Could you check a few things on this model? Use its own coordinates, in mm. Face numbers are marked on the shaded views. A direction names the side the tool comes from. Coordinates: 2 decimals unless noted, no trailing zeros. Loops run counter-clockwise (first coordinate to the right, second up) from the corner with the lowest first, then second, coordinate; pieces in that order, holes last.
1) Thinking about a two-plate mould opening in X: for the marked faces 1, 2, 3 and 4, which applies, released by +X, released by -X, zero draft, split by the parting line, or undercut?
2) For the marked faces 5, 6 and 7, which set-ups out of +Z, -Z, +X, -X, +Y, -Y let a thin tool reach every point of the face, with its end or its side?
3) Imagine slicing it at D-D on x = -197.5. Please give me the cut outline in (y, z), plus the area to 3 significant figures.
4) Imagine slicing it at C-C on y = -66. Please give me the cut outline in (x, z).
5) Imagine slicing it at A-A on y = 0. Please give me the cut outline in (x, z), plus the area to 3 significant figures.
6) Will these pins go through, and if not, where does the flat tip stop? P1, Ø9.5, axis at y = -12, z = 20, coming from the -X side; P2, Ø4, axis at x = -90.5, y = 101, coming from the -Z side; P3, Ø5, axis at y = -100.5, z = -15.5, coming from the +X side; P4, Ø24, axis at x = 0, y = 0, coming from the -Z side.
7) If I drill on line 1 along Z through (x, y) = (47.5, -89); line 2 along Y through (x, z) = (-156, -18); line 3 along X through (y, z) = (-44, 22.5), over which ranges is the centre line in solid material (lowest first)?
8) Imagine slicing it at B-B on x = -27. Please give me the cut outline in (y, z), plus the area to 3 significant figures.
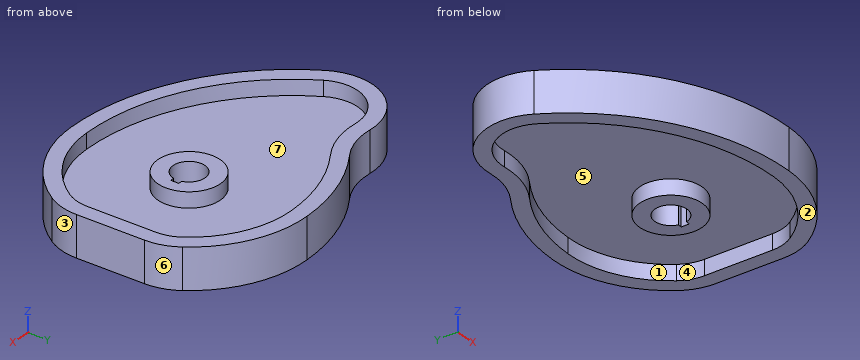
```python
from build123d import *

# Parameters (mm, degrees)
BOSS_EXTRUDE1_DEPTH   = 25.4
SKETCH1_R             = 39.05
BOSS_EXTRUDE1_2_DEPTH = 25.4
SKETCH1_3_R           = 39.05
BOSS_EXTRUDE2_DEPTH   = 6.35


with BuildPart() as part:
    # Sketch1 → Boss-Extrude1 (new, symmetric)
    with BuildSketch(Plane.XY):
        with BuildLine():
            ThreePointArc((133.35, 42.12), (130.375973078, 62.28554269), (121.707130955, 80.733987729))
            ThreePointArc((121.707130955, 80.733987729), (69.063027707, 128.689163118), (0, 146.05))
            ThreePointArc((0, 146.05), (-62.467080094, 137.090708669), (-119.897842805, 110.935164495))
            ThreePointArc((-119.897842805, 110.935164495), (-144.729719838, 100.277998184), (-171.672691668, 98.210734349))
            ThreePointArc((-171.672691668, 98.210734349), (-236.354801658, 66.713562108), (-238.919816081, -5.184058944))
            ThreePointArc((-238.919816081, -5.184058944), (-138.677586388, -108.211737191), (0, -146.05))
            ThreePointArc((0, -146.05), (69.063027707, -128.689163118), (121.707130955, -80.733987729))
            ThreePointArc((121.707130955, -80.733987729), (130.375973078, -62.28554269), (133.35, -42.12))
            Line((133.35, -42.12), (133.35, 42.12))
        make_face()
        with BuildLine():
            ThreePointArc((0, -127), (60.054806702, -111.903620102), (105.832287787, -70.20346759))
            ThreePointArc((105.832287787, -70.20346759), (112.137027627, -56.786145557), (114.3, -42.12))
            Line((114.3, -42.12), (114.3, 42.12))
            ThreePointArc((114.3, 42.12), (112.137027627, 56.786145557), (105.832287787, 70.20346759))
            ThreePointArc((105.832287787, 70.20346759), (60.054806702, 111.903620102), (0, 127))
            ThreePointArc((0, 127), (-57.112758943, 118.808647926), (-109.62088485, 94.895007539))
            ThreePointArc((-109.62088485, 94.895007539), (-140.183195045, 81.778495155), (-173.343775759, 79.234170436))
            ThreePointArc((-173.343775759, 79.234170436), (-220.385310297, 56.327136078), (-222.250775331, 4.037957131))
            ThreePointArc((-222.250775331, 4.037957131), (-129.002280352, -91.801650259), (0, -127))
        make_face(mode=Mode.SUBTRACT)
    extrude(amount=BOSS_EXTRUDE1_DEPTH, both=True)



with BuildPart() as body_2:
    # Sketch1 → Boss-Extrude1 2 (new, symmetric)
    with BuildSketch(Plane.XY):
        Circle(SKETCH1_R)
        with BuildLine():
            ThreePointArc((19.364916731, 5), (-20, 0), (19.364916731, -5))
            Line((19.364916731, -5), (24.364916731, -5))
            Line((24.364916731, -5), (24.364916731, 5))
            Line((24.364916731, 5), (19.364916731, 5))
        make_face(mode=Mode.SUBTRACT)
    extrude(amount=BOSS_EXTRUDE1_2_DEPTH, both=True)


with BuildPart() as part_1:
    add(part.part)

    add(body_2.part)  # Boss-Extrude2 merges body 2
    # Sketch1_3 → Boss-Extrude2 (add, symmetric)
    with BuildSketch(Plane.XY):
        with BuildLine():
            ThreePointArc((0, -127), (-129.002280352, -91.801650259), (-222.250775331, 4.037957131))
            ThreePointArc((-222.250775331, 4.037957131), (-220.385310297, 56.327136078), (-173.343775759, 79.234170436))
            ThreePointArc((-173.343775759, 79.234170436), (-140.183195045, 81.778495155), (-109.62088485, 94.895007539))
            ThreePointArc((-109.62088485, 94.895007539), (-57.112758943, 118.808647926), (0, 127))
            ThreePointArc((0, 127), (60.054806702, 111.903620102), (105.832287787, 70.20346759))
            ThreePointArc((105.832287787, 70.20346759), (112.137027627, 56.786145557), (114.3, 42.12))
            Line((114.3, 42.12), (114.3, -42.12))
            ThreePointArc((114.3, -42.12), (112.137027627, -56.786145557), (105.832287787, -70.20346759))
            ThreePointArc((105.832287787, -70.20346759), (60.054806702, -111.903620102), (0, -127))
        make_face()
        Circle(SKETCH1_3_R, mode=Mode.SUBTRACT)
    extrude(amount=BOSS_EXTRUDE2_DEPTH, both=True)


solid = part_1.part
```
Filled in:
1. face 1: undercut
1. face 2: zero draft
1. face 3: released by +X
1. face 4: undercut
2. face 5: -Z
2. face 6: +Z, -Z, +X, +Y
2. face 7: +Z
3. outline: (-61.55, -25.4) - (-32.72, -25.4) - (-32.72, -6.35) - (75.45, -6.35) - (75.45, -25.4) - (95.64, -25.4) - (95.64, 25.4) - (75.45, 25.4) - (75.45, 6.35) - (-32.72, 6.35) - (-32.72, 25.4) - (-61.55, 25.4) - close
3. area: 3,860 mm2
4. outline: (-193.15, -25.4) - (-165.13, -25.4) - (-165.13, -6.35) - (108.34, -6.35) - (108.34, -25.4) - (129.14, -25.4) - (129.14, 25.4) - (108.34, 25.4) - (108.34, 6.35) - (-165.13, 6.35) - (-165.13, 25.4) - (-193.15, 25.4) - close
5. outline: (-241.51, -25.4) - (-219.97, -25.4) - (-219.97, -6.35) - (-39.05, -6.35) - (-39.05, -25.4) - (-20, -25.4) - (-20, 25.4) - (-39.05, 25.4) - (-39.05, 6.35) - (-219.97, 6.35) - (-219.97, 25.4) - (-241.51, 25.4) - close; (24.36, -25.4) - (39.05, -25.4) - (39.05, -6.35) - (114.3, -6.35) - (114.3, -25.4) - (133.35, -25.4) - (133.35, 25.4) - (114.3, 25.4) - (114.3, 6.35) - (39.05, 6.35) - (39.05, 25.4) - (24.36, 25.4) - close
5. area: 7,030 mm2
6. P1: stops at x = -237.77
6. P2: stops at z = -6.35
6. P3: stops at x = 108.29
6. P4: passes through
7. line 1: z = -6.35 to 6.35
7. line 2: y = -97.1 to -73.45, 79.19 to 98.32
7. line 3: x = -212.87 to -187.81, 114.27 to 133.32
8. outline: (-144.71, -25.4) - (-125.56, -25.4) - (-125.56, -6.35) - (-28.21, -6.35) - (-28.21, -25.4) - (28.21, -25.4) - (28.21, -6.35) - (125.2, -6.35) - (125.2, -25.4) - (144.4, -25.4) - (144.4, 25.4) - (125.2, 25.4) - (125.2, 6.35) - (28.21, 6.35) - (28.21, 25.4) - (-28.21, 25.4) - (-28.21, 6.35) - (-125.56, 6.35) - (-125.56, 25.4) - (-144.71, 25.4) - close
8. area: 7,280 mm2
